Autodesk Inventor part; units mm, degrees
ref_plane "YZ Plane" through (0, 0, 0) normal (1, 0, 0) x (0, 1, 0)
ref_plane "XZ Plane" through (0, 0, 0) normal (0, 1, 0) x (-1, 0, 0)
ref_plane "XY Plane" through (0, 0, 0) normal (0, 0, 1) x (1, 0, 0)
sketch "Sketch1" plane through (0, 0, 0) normal (0, 0, 1) x (1, 0, 0)
  line L0 (0, 0) -> (25.4, 0)
  line L1 (25.4, 0) -> (25.4, 50.8)
  line L2 (25.4, 50.8) -> (0, 50.8)
  line L3 (0, 50.8) -> (0, 0)
  line L4 (22.86, 48.26) -> (2.54, 48.26)
  line L5 (2.54, 48.26) -> (2.54, 2.54)
  line L6 (2.54, 2.54) -> (22.86, 2.54)
  line L7 (22.86, 2.54) -> (22.86, 48.26)
  dimension "d0" = 50.8
  dimension "d1" = 25.4
  dimension "d2" = 2.54
  dimension "d3" = 2.54
  dimension "d4" = 2.54
  dimension "d5" = 2.54
extrude "Extrusion1" add sketch "Sketch1" along normal blind 203.2
sketch "Sketch2" plane through (25.4, 0, 0) normal (1, 0, 0) x (0, 0, -1)
  circle A0 centre (-12.7, 12.7) radius 2.5797
  circle A1 centre (-63.5, 12.7) radius 2.5797
  circle A2 centre (-38.1, 12.7) radius 2.5797
  line L0 (0, 2.54) -> (-203.2, 2.54)
  line L1 (0, 0) -> (-203.2, 0)
  line L2 (0, 0) -> (0, 50.8)
  line L3 (-203.2, 0) -> (-203.2, 50.8)
  dimension "d8" = 5.1594
  dimension "d10" = 5.1594
  dimension "d11" = 5.1594
  dimension "d12" = 12.7
  dimension "d13" = 12.7
  dimension "d14" = 12.7
  dimension "d16" = 12.7
  dimension "d18" = 38.1
  dimension "d21" = 25.4
extrude "Extrusion2" cut sketch "Sketch2" against normal blind 203.2 contours A0 | A1 | A2
sketch "Sketch3" plane through (25.4, 0, 0) normal (1, 0, 0) x (0, 0, -1)
  circle A0 centre (-138.2776, 12.7) radius 2.5797
  line L0 (-203.2, 0) -> (-203.2, 50.8)
  line L1 (0, 0) -> (-203.2, 0)
  dimension "d24" = 5.1594
  dimension "d25" = 64.9224
  dimension "d26" = 12.7
extrude "Extrusion3" cut sketch "Sketch3" against normal blind 203.2
sketch "Sketch4" plane through (0, 0, 0) normal (-1, 0, 0) x (0, 0, 1)
  circle A0 centre (177.8, 25.4) radius 14.2875
  line L0 (203.2, 50.8) -> (203.2, 0)
  line L1 (0, 0) -> (203.2, 0)
  dimension "d29" = 28.575
  dimension "d31" = 25.4
  dimension "d32" = 25.4
extrude "Extrusion4" cut sketch "Sketch4" against normal blind 25.4
equation "\"d3\" = d2"
equation "\"d4\" = d2"
equation "\"d5\" = d2"
properties part number "1x2"
Source: CAD feature listing. Evaluate the final solid. Frame: model axes, mm. A direction names the side the tool comes from. Coordinates: 2 decimals unless noted, no trailing zeros. Loops run counter-clockwise (first coordinate to the right, second up) from the corner with the lowest first, then second, coordinate; pieces in that order, holes last. Notation, with made-up numbers: (-7, 80.25) - (-1, 80.25) arc R20 cw to (-1, 113.25) - close; hole circle Ø8 at (-17, 18.25). An arc over 180 degrees is marked (long way). One line per item, written item: value. Start each with the question number.
1. Mould query, pull axis X, two halves, no side actions, for faces 3 (the flat face through (25.4, 25, 100)), 4 (the flat face through (0, 26, 100)), 5 (the cylindrical face through (24.148, 12.813, 40.677)), 6 (the flat face through (2.54, 26, 100)). Classes: pulls with the +X half, pulls with the -X half, needs draft (parallel to the pull), parting line crosses it, or undercut.
2. Section D-D (z = 38.1). Return the cut outline in (x, y), and give its area (3 significant figures).
3. Section C-C (x = 17.5). Return the cut outline in (y, z), and give its area (3 significant figures).
4. Ray query, L1, parallel to Y at x = 9.75, z = 69; L2, parallel to X at y = 27.5, z = 131; L3, parallel to Y at x = 2, z = 38.1. Return the intervals inside material, ascending.
5. Section B-B (y = 43). Return the cut outline in (x, z).
6. Set-up query: faces 1 (the cylindrical face through (1.288, 12.813, 40.677)), 2 (the flat face through (22.86, 25, 100)). Return all of +Z, -Z, +X, -X, +Y, -Y with unobstructed straight access to the full face (end or side cutting, diameter ignored); none if empty.
7. Section A-A (z = 146). Return the cut outline in (x, y), and give its area (3 significant figures).
8. Contact query for flat-ended pins moving along their axis: P1, Ø4, axis at y = 12.7, z = 12.7, coming from the +X side; P2, Ø8, axis at x = 11.5, z = 82.5, coming from the -Y side. Output: stop coordinate, or through.
Verdict:
1. face 3: pulls with the +X half
1. face 4: pulls with the -X half
1. face 5: needs draft
1. face 6: undercut
2. outline: (0, 0) - (25.4, 0) - (25.4, 10.12) - (22.86, 10.12) - (22.86, 2.54) - (2.54, 2.54) - (2.54, 10.12) - (0, 10.12) - close; (0, 15.28) - (2.54, 15.28) - (2.54, 48.26) - (22.86, 48.26) - (22.86, 15.28) - (25.4, 15.28) - (25.4, 50.8) - (0, 50.8) - close
2. area: 335 mm2
3. outline: (0, 0) - (2.54, 0) - (2.54, 203.2) - (0, 203.2) - close; (48.26, 0) - (50.8, 0) - (50.8, 203.2) - (48.26, 203.2) - close
3. area: 1,030 mm2
4. L1: y = 0 to 2.54, 48.26 to 50.8
4. L2: x = 0 to 2.54, 22.86 to 25.4
4. L3: y = 0 to 10.12, 15.28 to 50.8
5. outline: (0, 0) - (2.54, 0) - (2.54, 203.2) - (0, 203.2) - close; (22.86, 0) - (25.4, 0) - (25.4, 203.2) - (22.86, 203.2) - close
6. face 1: +X, -X
6. face 2: +Z, -Z
7. outline: (0, 0) - (25.4, 0) - (25.4, 50.8) - (0, 50.8) - close; hole (2.54, 2.54) - (22.86, 2.54) - (22.86, 48.26) - (2.54, 48.26) - close
7. area: 361 mm2
8. P1: passes through
8. P2: stops at y = 0
